Build history of the part. All positions in model axes, mm. Round coordinates to 2 decimals unless told otherwise and drop trailing zeros. Loops run counter-clockwise (first coordinate to the right, second up) from the corner with the lowest first, then second, coordinate; pieces in that order, holes last. Notation, with made-up numbers: M 8,-2 L 46,-2 A36 ccw 46,35 Z; hole C 69,-28.75 d4. An arc over 180 degrees is marked long. One line per item, written item: value.
```python
from build123d import *

# Parameters (mm, degrees)
F1_DEPTH = 17.8562


with BuildPart() as f1:
    # F0 (on Front) → F1 (new body)
    with BuildSketch(Plane.XZ):
        with BuildLine():
            Line((254, 471.312474), (-254, 471.312474))
            Line((-254, 471.312474), (-254, -341.487526))
            Line((-254, -341.487526), (-177.8, -341.487526))
            Line((-177.8, -341.487526), (-154.149531, 320.725604))
            ThreePointArc((-154.149531, 320.725604), (-138.65606, 355.468917), (-103.381898, 369.712474))
            Line((-103.381898, 369.712474), (103.381898, 369.712474))
            ThreePointArc((103.381898, 369.712474), (138.65606, 355.468917), (154.149531, 320.725604))
            Line((154.149531, 320.725604), (177.8, -341.487526))
            Line((177.8, -341.487526), (254, -341.487526))
            Line((254, -341.487526), (254, 471.312474))
        make_face()
    extrude(amount=F1_DEPTH)


solid = f1.part
```
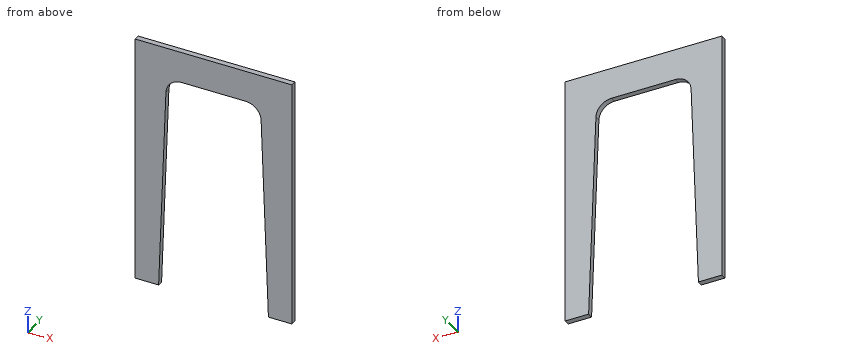
Item 1: Slice it at B-B, the plane y = -11.75. Give the cut face in (x, z), and give its area (3 significant figures).
Check values:
outline: M -254,-341.49 L -177.8,-341.49 L -154.15,320.73 A50.8 cw -103.38,369.71 L 103.38,369.71 A50.8 cw 154.15,320.73 L 177.8,-341.49 L 254,-341.49 L 254,471.31 L -254,471.31 Z
area: 179,000 mm2
Item 2: Wall check: line 1 along Z through (x, y) = (101.5, -12.5); line 2 along X through (y, z) = (-13, -236); line 3 along X through (y, z) = (-16.75, -35). Give the ranges that are in metal, low to high.
Check values:
line 1: z = 369.71 to 471.31
line 2: x = -254 to -174.03, 174.03 to 254
line 3: x = -254 to -166.85, 166.85 to 254
Item 3: Slice it at C-C, the plane z = 246.5. Give the cut face in (x, y), and give its area (3 significant figures).
Check values:
outline: M -254,-17.86 L -156.8,-17.86 L -156.8,0 L -254,0 Z; M 156.8,-17.86 L 254,-17.86 L 254,0 L 156.8,0 Z
area: 3,470 mm2
Item 4: Slice it at A-A, the plane z = 143. Give the cut face in (x, y).
Check values:
outline: M -254,-17.86 L -160.5,-17.86 L -160.5,0 L -254,0 Z; M 160.5,-17.86 L 254,-17.86 L 254,0 L 160.5,0 Z
Item 5: Slice it at D-D, the plane x = 20. Give the cut face in (y, z).
Check values:
outline: M -17.86,369.71 L 0,369.71 L 0,471.31 L -17.86,471.31 Z
Item 6: Drop a flat-ended pin along its axis: P1, Ø1.5, axis at x = -100, y = -6, coming from the -Z side. Give the stop position or say it passes through.
Check values:
P1: stops at z = 369.71
